```python
from build123d import *

# Parameters (mm, degrees)
F0_W           = 711.2
F0_H           = 406.4
F1_DEPTH       = 19.05
F2_W           = 222.25
F2_H           = 19.05
F3_DEPTH       = 0.00254
F4_R           = 12.7
F5_R           = 12.7
F7_D           = 1.190625
F7_CSINK_D     = 6.35
F7_CSINK_ANGLE = 90


with BuildPart() as f1:
    # F0 (on Top) → F1 (new body)
    with BuildSketch(Plane.XY):
        Rectangle(F0_W, F0_H)
    extrude(amount=F1_DEPTH)

    # F2 (on face) → F3 (join)
    with BuildSketch(Plane.XZ.offset(203.2)):
        with Locations((-22.225, 9.525)):
            Rectangle(F2_W, F2_H)
    extrude(amount=F3_DEPTH)

    # F4
    f4_edges = [f1.edges().sort_by_distance(p)[0] for p in [
        (-244.475, -203.2, 19.05),
        (-355.6, 0, 19.05),
        (222.25, -203.2, 19.05),
        (355.6, 0, 19.05),
        (0, 203.2, 19.05),
    ]]
    fillet(f4_edges, radius=F4_R)

    # F5
    f5_edges = [f1.edges().sort_by_distance(p)[0] for p in [
        (88.9, -203.20127, 19.05),
        (-133.35, -203.20127, 19.05),
    ]]
    fillet(f5_edges, radius=F5_R)

    # F7 (through all)
    with Locations(Plane(origin=(0, 0, 0), x_dir=(1, 0, 0), z_dir=(0, 0, -1))):
        with Locations((190.5, -161.925), (190.5, 161.925), (-190.5, -161.925), (-190.5, 161.925)):
            CounterSinkHole(F7_D / 2, F7_CSINK_D / 2, counter_sink_angle=F7_CSINK_ANGLE)


solid = f1.part
```
Input: part model. Units: mm. Frame: model coordinates. A direction names the side the tool comes from. Give positions to 0.01 mm unless a question says otherwise; leave off trailing zeros. Loops run counter-clockwise (first coordinate to the right, second up) from the corner with the lowest first, then second, coordinate; pieces in that order, holes last. Notation, with made-up numbers: (75, -1) -> (101, -1) arc R23 cw to (101, 14) -> close; hole circle Ø11 at (55.5, 49.5). An arc over 180 degrees is marked (long way). Use a Markdown table: item, result.
Q1. Ray query, probe 1 along Y at (x, z) = (190.5, 9.25); probe 2 along Y at (x, z) = (-190.5, 15.75); probe 3 along Y at (x, z) = (-203, 3.75). Return the intervals inside material, ascending. Write a range as from..to.
Entries:
| item | result |
|---|---|
| probe 1 | y = -202.86..-162.52, -161.33..161.33, 162.52..202.86 |
| probe 2 | y = -199.04..-162.52, -161.33..161.33, 162.52..199.04 |
| probe 3 | y = -203.2..203.2 |
Q2. First-contact query: P1, Ø0.7, axis at x = 190.5, y = 161.925, coming from the -Z side; P2, Ø6, axis at y = -34, z = 14, coming from the +X side; P3, Ø6, axis at x = 211, z = 3, coming from the -Y side; P4, Ø1, axis at y = -125, z = 12, coming from the +X side. Flat tips, straight axial feed; report the tip coordinate or a pass-through.
Entries:
| item | result |
|---|---|
| P1 | passes through |
| P2 | stops at x = 354.72 |
| P3 | stops at y = -203.2 |
| P4 | stops at x = 354.51 |
Q3. Access query for faces 1 (the cylindrical face through (-125.89, -199.59, 17.92)), 2 (the cylindrical face through (-351.98, 2.84, 15.23)), 3 (the cylindrical face through (217.86, -199.38, 15.43)). Directions: +Z, -Z, +X, -X, +Y, -Y. A direction counts if a zero-diameter tool reaches every point of the face in a straight line with its end or side. Return the directions, or none.
Entries:
| item | result |
|---|---|
| face 1 | +Z, -X, -Y |
| face 2 | +Z, -X, +Y, -Y |
| face 3 | +Z, +X, -Y |
Q4. Section query A-A, the plane z = 14.25. Return the cut outline in (x, y) (3 decimals), plus the area to 3 significant figures.
Entries:
| item | result |
|---|---|
| outline | (-352.844, -200.444) -> (-130.594, -200.444) -> (-130.594, -203.203) -> (86.144, -203.203) -> (86.144, -200.444) -> (352.844, -200.444) -> (352.844, 200.444) -> (-352.844, 200.444) -> close; hole circle Ø1.191 at (-190.5, -161.925); hole circle Ø1.191 at (-190.5, 161.925); hole circle Ø1.191 at (190.5, -161.925); hole circle Ø1.191 at (190.5, 161.925) |
| area | 283,000 mm² |
